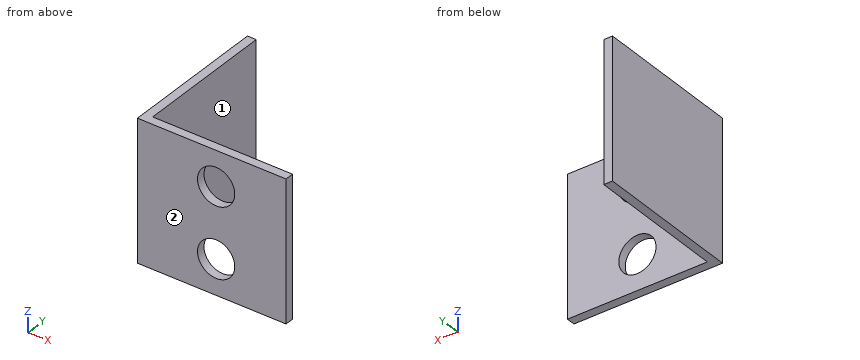
```python
from build123d import *

# Parameters (mm, degrees)
BOSS_EXTRUDE1_DEPTH     = 25.4
F_1_4_CLEARANCE_HOLE1_D = 6.7564


with BuildPart() as part:
    # Sketch1 → Boss-Extrude1 (new body)
    with BuildSketch(Plane.XY):
        Polygon((0, 0), (0, 25.4), (-1.5875, 25.4), (-1.5875, -1.5875), (25.4, -1.5875), (25.4, 0), align=None)
    extrude(amount=BOSS_EXTRUDE1_DEPTH)

    # 1/4 Clearance Hole1 (through all)
    with Locations(Plane(origin=(12.7, 0, 19.05), x_dir=(1, 0, 0), z_dir=(0, 1, 0))):
        with Locations((0, 0), (0, 12.7)):
            Hole(F_1_4_CLEARANCE_HOLE1_D / 2)


solid = part.part
```
The model under review builds one solid part; all positions refer to its coordinate system, in mm. Face numbers are marked on the shaded views. A direction names the side the tool comes from. Coordinates: 2 decimals unless noted, no trailing zeros. Write each loop counter-clockwise with the first axis right and the second up, starting at its lowest first coordinate (ties: lowest second). Pieces come first, ordered by that corner, then holes.
1) Clearance check with flat-ended pins moving along their axes: pin 1 Ø5 at (x, z) = (20.5, 16) entering from +Y; pin 2 Ø8 at (x, z) = (12.7, 6.35) entering from -Y; pin 3 Ø7.5 at (y, z) = (12.5, 13) entering from +X. State where each tip first meets the part, or that it passes through.
2) We need section B-B on z = 21.75. State the section outline as (x, y) points, then the cut area to 3 significant figures.
3) To check wall thickness, follow probe 1 along Z at (x, y) = (12.7, -1.15); probe 2 along X at (y, z) = (-0.8, 19.05); probe 3 along Y at (x, z) = (2.75, 19.75). State the ranges of each line that lie inside material, in increasing order.
4) Machinability: for the marked faces 1 and 2, which of the approach directions +Z, -Z, +X, -X, +Y, -Y give a long, thin tool a straight path to every point of the face, cutting with its end or side? Answer none if there is none.
5) We need section D-D on x = 6.75. State the section outline as (y, z) points, then the cut area to 3 significant figures.
6) We need section A-A on x = 12.7. State the section outline as (y, z) points, then the cut area to 3 significant figures.
7) We need section C-C on z = 13.5. State the section outline as (x, y) points.
Answer list:
1. pin 1: stops at y = 0
1. pin 2: stops at y = -1.59
1. pin 3: stops at x = 0
2. outline: (-1.59, -1.59) - (10.67, -1.59) - (10.67, 0) - (0, 0) - (0, 25.4) - (-1.59, 25.4) - close; (14.73, -1.59) - (25.4, -1.59) - (25.4, 0) - (14.73, 0) - close
2. area: 76.7 mm2
3. probe 1: z = 0 to 2.97, 9.73 to 15.67, 22.43 to 25.4
3. probe 2: x = -1.59 to 9.32, 16.08 to 25.4
3. probe 3: y = -1.59 to 0
4. face 1: +Z, -Z, +X, +Y
4. face 2: +Z, -Z, +X, -X, -Y
5. outline: (-1.59, 0) - (0, 0) - (0, 25.4) - (-1.59, 25.4) - close
5. area: 40.3 mm2
6. outline: (-1.59, 0) - (0, 0) - (0, 2.97) - (-1.59, 2.97) - close; (-1.59, 9.73) - (0, 9.73) - (0, 15.67) - (-1.59, 15.67) - close; (-1.59, 22.43) - (0, 22.43) - (0, 25.4) - (-1.59, 25.4) - close
6. area: 18.9 mm2
7. outline: (-1.59, -1.59) - (25.4, -1.59) - (25.4, 0) - (0, 0) - (0, 25.4) - (-1.59, 25.4) - close
